The model under review builds one solid part; all positions refer to its coordinate system, in mm. A direction names the side the tool comes from. Coordinates: 2 decimals unless noted, no trailing zeros. Write each loop counter-clockwise with the first axis right and the second up, starting at its lowest first coordinate (ties: lowest second). Pieces come first, ordered by that corner, then holes. Notation, with made-up numbers: M 73,-9 L 131,-9 A24 cw 131,22 Z; hole C -12.75,-21.75 d1. An arc over 180 degrees is marked long. Answer as a JSON object with one key per item and string values.
```python
from build123d import *

# Parameters (mm, degrees)
SKETCH1_W              = 1930.4
SKETCH1_H              = 1447.8
BOSS_EXTRUDE1_DEPTH    = 1549.4
CUT_EXTRUDE1_DEPTH     = 1447.8
CUT_EXTRUDE2_DEPTH     = 25.4
CUT_EXTRUDE3_START     = -1447.8
CUT_EXTRUDE3_OUTLINE_W = 1371.6
CUT_EXTRUDE3_OUTLINE_H = 1447.8
CUT_EXTRUDE3_DEPTH     = 25.4
SKETCH4_W              = 1346.2
SKETCH4_H              = 939.8
CUT_EXTRUDE4_DEPTH     = 25.4
SKETCH5_W              = 1346.2
SKETCH5_H              = 1447.8
CUT_EXTRUDE5_DEPTH     = 25.4


# Read off the part's stored shape, not the designer's step: Cut-Extrude3
with BuildPart() as part:
    # Sketch1 → Boss-Extrude1 (new body)
    with BuildSketch(Plane(origin=(0, 0, 0), x_dir=(1, 0, 0), z_dir=(0, 1, 0))):
        Rectangle(SKETCH1_W, SKETCH1_H)
    extrude(amount=BOSS_EXTRUDE1_DEPTH)

    # Sketch2 → Cut-Extrude1 (cut)
    with BuildSketch(Plane.XY.offset(723.9)):
        Polygon((-965.2, 0), (-508, 0), (-508, 50.8), (-965.2, 508), align=None)
    extrude(amount=-CUT_EXTRUDE1_DEPTH, mode=Mode.SUBTRACT)

    # Sketch3 → Cut-Extrude2 (cut)
    with BuildSketch(Plane.XY.offset(723.9)):
        Polygon((-914.4, 1498.6), (-914.4, 529.042048969), (-508, 122.642048969), (-508, 1498.6), align=None)
        Polygon((-457.2, 71.842048969), (-457.2, 50.8), (914.4, 50.8), (914.4, 1498.6), (-457.2, 1498.6), align=None)
    extrude(amount=-CUT_EXTRUDE2_DEPTH, mode=Mode.SUBTRACT)

    # Cut-Extrude3 outline → Cut-Extrude3 (cut)
    with BuildSketch(Plane.XY.offset(723.9).offset(CUT_EXTRUDE3_START)):
        Polygon((-508, 122.642048969), (-508, 1498.6), (-914.4, 1498.6), (-914.4, 529.042048969), align=None)
        with Locations((228.6, 774.7)):
            Rectangle(CUT_EXTRUDE3_OUTLINE_W, CUT_EXTRUDE3_OUTLINE_H)
    extrude(amount=CUT_EXTRUDE3_DEPTH, mode=Mode.SUBTRACT)

    # Sketch4 → Cut-Extrude4 (cut)
    with BuildSketch(Plane.ZY.offset(965.2)):
        with Locations((0, 1028.7)):
            Rectangle(SKETCH4_W, SKETCH4_H)
    extrude(amount=-CUT_EXTRUDE4_DEPTH, mode=Mode.SUBTRACT)

    # Sketch5 → Cut-Extrude5 (cut)
    with BuildSketch(Plane(origin=(965.2, 0, 0), x_dir=(0, 0, -1), z_dir=(1, 0, 0))):
        with Locations((0, 774.7)):
            Rectangle(SKETCH5_W, SKETCH5_H)
    extrude(amount=-CUT_EXTRUDE5_DEPTH, mode=Mode.SUBTRACT)


solid = part.part
```
(1) Add section A-A on z = -81. Give the boundary of the cut face in (x, y).
Results list:
{"outline": "M -965.2,508 L -508,50.8 L -508,0 L 965.2,0 L 965.2,50.8 L 939.8,50.8 L 939.8,1498.6 L 965.2,1498.6 L 965.2,1549.4 L -965.2,1549.4 L -965.2,1498.6 L -939.8,1498.6 L -939.8,558.8 L -965.2,558.8 Z"}
(2) For pin 1 Ø7.5 at (x, z) = (137.5, -710) entering from -Y; pin 2 Ø6 at (y, z) = (214.5, -155) entering from +X; pin 3 Ø4 at (y, z) = (244, -408) entering from -X; pin 4 Ø12 at (y, z) = (1108.5, 301) entering from -X, all flat-tipped, find the tip position at first contact; note any pin that passes through.
Results list:
{"pin 1": "y = 0", "pin 2": "x = 939.8", "pin 3": "x = -703.2", "pin 4": "x = -939.8"}
(3) Wall thickness on line 1 along Z through (x, y) = (544.5, 1183); line 2 along X through (y, z) = (846.5, 480.5); line 3 along X through (y, z) = (534, -414): over which ranges is each line inside the solid? List them lowest first. Write a range as from..to.
Results list:
{"line 1": "-698.5..698.5", "line 2": "-939.8..939.8", "line 3": "-965.2..939.8"}
(4) Add section C-C on y = 1049. Give the boundary of the cut face in (x, z).
Results list:
{"outline": "M -965.2,-723.9 L -914.4,-723.9 L -914.4,-698.5 L -508,-698.5 L -508,-723.9 L -457.2,-723.9 L -457.2,-698.5 L 914.4,-698.5 L 914.4,-723.9 L 965.2,-723.9 L 965.2,-673.1 L 939.8,-673.1 L 939.8,673.1 L 965.2,673.1 L 965.2,723.9 L 914.4,723.9 L 914.4,698.5 L -457.2,698.5 L -457.2,723.9 L -508,723.9 L -508,698.5 L -914.4,698.5 L -914.4,723.9 L -965.2,723.9 L -965.2,673.1 L -939.8,673.1 L -939.8,-673.1 L -965.2,-673.1 Z"}
(5) Add section B-B on x = 738.5. Give the boundary of the cut face in (y, z).
Results list:
{"outline": "M 0,-723.9 L 50.8,-723.9 L 50.8,-698.5 L 1498.6,-698.5 L 1498.6,-723.9 L 1549.4,-723.9 L 1549.4,723.9 L 1498.6,723.9 L 1498.6,698.5 L 50.8,698.5 L 50.8,723.9 L 0,723.9 Z"}
(6) For faces 4 (the face through (219, 785, 698.5)), 5 (the face through (-714, 973, -698.5)), 6 (the face through (939.8, 785, 9)), 7 (the face through (-508, 25, 10)), list the 3-axis set-ups (+Z, -Z, +X, -X, +Y, -Y) from which the entire face can be reached by the end or side of a thin tool; tool diameter is ignored.
Results list:
{"face 4": "+Z", "face 5": "-Z", "face 6": "+X", "face 7": "+Z, -Z, -X, -Y"}
(7) Draft analysis for pull direction Y (two halves, no side actions). For faces 1 (the face through (218, 0, -10)), 2 (the face through (-965.2, 1528, 57)), 3 (the face through (-939.8, 1035, -9)), state which applies: released by +Y, released by -Y, zero draft, split by the parting line, or undercut.
Results list:
{"face 1": "released by -Y", "face 2": "zero draft", "face 3": "undercut"}
